```python
from build123d import *

# Parameters (mm, degrees)
SKETCH1_R                 = 4.5
SKETCH1_R_2               = 2.95
BOSS_EXTRUDE2_DEPTH       = 3.6
BOSS_EXTRUDE3_START       = 1.6
SKETCH1_4_R               = 9.975
SKETCH1_4_R_2             = 1.6
BOSS_EXTRUDE3_DEPTH       = 2.5
SKETCH1_6_R               = 2.95
CUT_EXTRUDE1_DEPTH        = 1.6
M3X0_5_TAPPED_HOLE1_D     = 3
M3X0_5_TAPPED_HOLE1_DEPTH = 2.5


with BuildPart() as part:
    # Sketch1 → Boss-Extrude2 (new body)
    with BuildSketch(Plane.XY):
        Circle(SKETCH1_R)
        Circle(SKETCH1_R_2, mode=Mode.SUBTRACT)
    extrude(amount=BOSS_EXTRUDE2_DEPTH)

    # Sketch1<4> → Boss-Extrude3 (add)
    with BuildSketch(Plane.XY.offset(BOSS_EXTRUDE3_START)):
        Circle(SKETCH1_4_R)
        Circle(SKETCH1_4_R_2, mode=Mode.SUBTRACT)
    extrude(amount=-BOSS_EXTRUDE3_DEPTH)

    # Sketch1<6> → Cut-Extrude1 (cut)
    with BuildSketch(Plane.XY):
        Circle(SKETCH1_6_R)
    extrude(amount=CUT_EXTRUDE1_DEPTH, mode=Mode.SUBTRACT)

    # M3x0.5 Tapped Hole1
    with Locations(Plane(origin=(0, 0, -0.9), x_dir=(-1, 0, 0), z_dir=(0, 0, -1))):
        with Locations((0, 7), (7, 0), (0, -7), (-7, 0)):
            Hole(M3X0_5_TAPPED_HOLE1_D / 2, depth=M3X0_5_TAPPED_HOLE1_DEPTH)


solid = part.part
```
Part model, mm, in its own coordinate system. A direction names the side the tool comes from. Round coordinates to 2 decimals unless told otherwise and drop trailing zeros. Loops run counter-clockwise (first coordinate to the right, second up) from the corner with the lowest first, then second, coordinate; pieces in that order, holes last. Notation, with made-up numbers: (-14, 32.5) -> (-2, 32.5) arc R14 cw to (-2, 58.5) -> close; hole circle Ø11 at (66.25, 63). An arc over 180 degrees is marked (long way). Use a Markdown table: item, result.
1) Cut at D-D, the plane x = 7. List the corners of the cut face in (y, z).
The answers:
| item | result |
|---|---|
| outline | (-7.11, -0.9) -> (-1.5, -0.9) -> (-1.5, 1.6) -> (-7.11, 1.6) -> close; (1.5, -0.9) -> (7.11, -0.9) -> (7.11, 1.6) -> (1.5, 1.6) -> close |
2) Drop flat-ended pins along their axis: pin 1 Ø1 at (y, z) = (6, -0.5) entering from -X; pin 2 Ø1.8 at (x, y) = (-7, 0) entering from -Z; pin 3 Ø1 at (x, z) = (0, 2.5) entering from -Y; pin 4 Ø1 at (y, z) = (-7, 2) entering from -X. Give the stop position or say it passes through.
The answers:
| item | result |
|---|---|
| pin 1 | stops at x = -8.32 |
| pin 2 | passes through |
| pin 3 | stops at y = -4.5 |
| pin 4 | stops at x = -7.39 |
3) Tool access for faces 4 (the cylindrical face through (-1.27, -0.97, -0.44)), 5 (the cylindrical face through (-0.59, 4.46, 2.59)): list every direction of +Z, -Z, +X, -X, +Y, -Y with a clear straight run to the whole face (end or side of a thin tool).
The answers:
| item | result |
|---|---|
| face 4 | +Z, -Z |
| face 5 | +Z |
4) Probe line 1 (Y direction, x = 0, z = -0.35) (3 decimals); line 2 (Y direction, x = 0, z = 0.5) (3 decimals); line 3 (X direction, y = -1.25, z = 1.25). List the from-to ranges inside material, lowest first. Write a range as [from, to].
The answers:
| item | result |
|---|---|
| line 1 | y = [-9.975, -8.5], [-5.5, -1.6], [1.6, 5.5], [8.5, 9.975] |
| line 2 | y = [-9.975, -8.5], [-5.5, -2.95], [2.95, 5.5], [8.5, 9.975] |
| line 3 | x = [-9.9, -7.83], [-6.17, -2.67], [2.67, 6.17], [7.83, 9.9] |
5) Cut at A-A, the plane y = 0. List the corners of the cut face in (x, z) (3 decimals).
The answers:
| item | result |
|---|---|
| outline | (-9.975, -0.9) -> (-8.5, -0.9) -> (-8.5, 1.6) -> (-9.975, 1.6) -> close; (-5.5, -0.9) -> (-1.6, -0.9) -> (-1.6, 0) -> (-2.95, 0) -> (-2.95, 3.6) -> (-4.5, 3.6) -> (-4.5, 1.6) -> (-5.5, 1.6) -> close; (1.6, -0.9) -> (5.5, -0.9) -> (5.5, 1.6) -> (4.5, 1.6) -> (4.5, 3.6) -> (2.95, 3.6) -> (2.95, 0) -> (1.6, 0) -> close; (8.5, -0.9) -> (9.975, -0.9) -> (9.975, 1.6) -> (8.5, 1.6) -> close |
6) Pull direction Y, two halves, no side cores. Call faces 1 (the cylindrical face through (-0.325, 5.536, 0.368)), 2 (the flat face through (0, -2, -0.9)), 3 (the cylindrical face through (9.514, 2.996, 0.368)): pulls with the +Y half, pulls with the -Y half, needs draft (parallel to the pull), parting line crosses it, or undercut.
The answers:
| item | result |
|---|---|
| face 1 | undercut |
| face 2 | needs draft |
| face 3 | parting line crosses it |
7) Cut at C-C, the plane z = 1.15. List the corners of the cut face in (x, y) (3 decimals).
The answers:
| item | result |
|---|---|
| outline | circle Ø19.95 at (0, 0); hole circle Ø3 at (-7, 0); hole circle Ø5.9 at (0, 0); hole circle Ø3 at (0, -7); hole circle Ø3 at (0, 7); hole circle Ø3 at (7, 0) |
